Source: three-view drawing plus pictorial views. Frame: mm from the lowest corner of the part. A direction names the side the tool comes from. Give positions to 0.01 mm unless a question says otherwise; leave off trailing zeros. Loops run counter-clockwise (first coordinate to the right, second up) from the corner with the lowest first, then second, coordinate; pieces in that order, holes last. Notation, with made-up numbers: M 42,34 L 95,34 A24 cw 95,63 Z; hole C -1.75,-8 d11. An arc over 180 degrees is marked long. Write item = value, one per line.
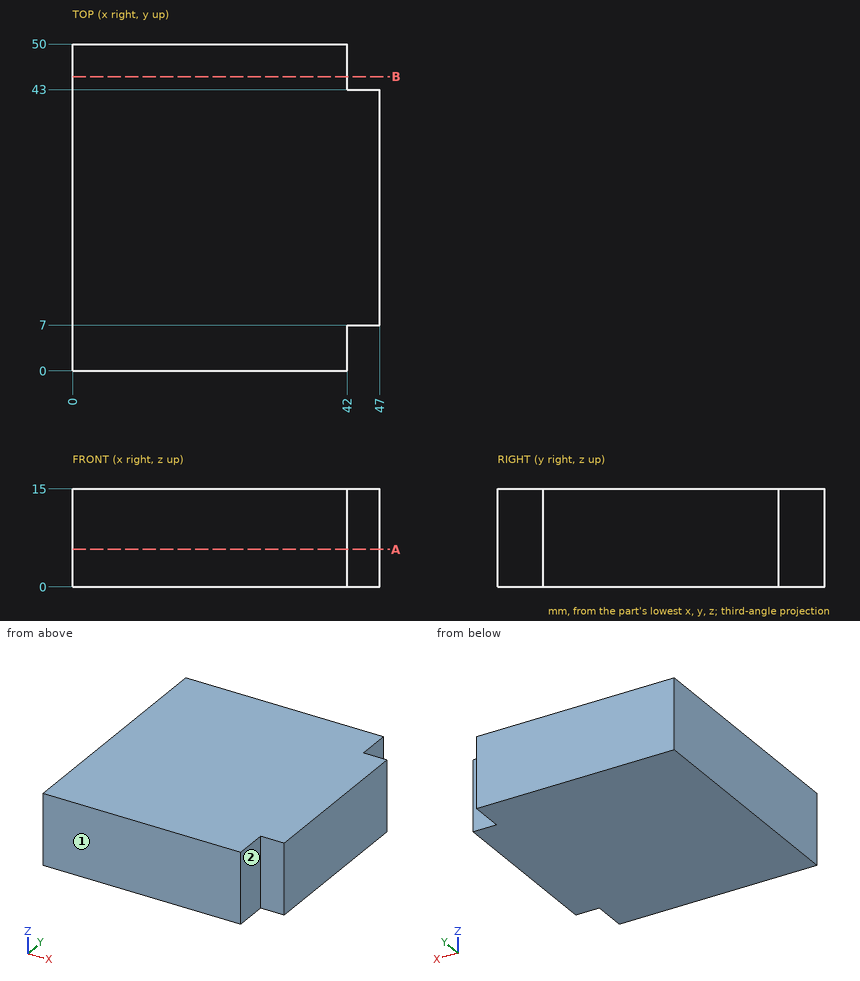
1. Material intervals for probe 1 along X at (y, z) = (47.5, 11.25); probe 2 along Y at (x, z) = (45, 2.5), sorted ascending. Write a range as from..to.
Derived:
probe_1 = 0..42
probe_2 = 7..43
2. First-contact query: pin 1 Ø2.5 at (x, z) = (45.5, 4.5) entering from +Y; pin 2 Ø5.5 at (y, z) = (46, 7) entering from +X. Flat tips, straight axial feed; report the tip coordinate or a pass-through.
Derived:
pin_1 = 43
pin_2 = 42
3. Cut plane A-A, the plane z = 5.75. Return the cut outline in (x, y).
Derived:
outline = M 0,0 L 42,0 L 42,7 L 47,7 L 47,43 L 42,43 L 42,50 L 0,50 Z
4. Cut plane B-B, the plane y = 45. Return the cut outline in (x, z).
Derived:
outline = M 0,0 L 42,0 L 42,15 L 0,15 Z
5. Reachability of the marked faces 1 and 2 from +Z, -Z, +X, -X, +Y, -Y: full face, straight path, thin tool, end or side. Return the list, or none.
Derived:
face_1 = +Z, -Z, +X, -X, -Y
face_2 = +Z, -Z, +X, -Y
